Model file for the job. Use its own axes, mm. A direction names the side the tool comes from. Coordinates: 2 decimals unless noted, no trailing zeros. Write each loop counter-clockwise with the first axis right and the second up, starting at its lowest first coordinate (ties: lowest second). Pieces come first, ordered by that corner, then holes.
Q1. Pull direction Y, two halves, no side cores. Call faces 5 (the flat face through (-10, -373.999, 48)), 6 (the flat face through (-10, -384.162, 52)), 7 (the flat face through (336, 19.556, 11)): released by +Y, released by -Y, zero draft, split by the parting line, or undercut.
Q2. Band-saw the part on D-D, the plane y = -91.5. Write the cut outline in (x, z).
Q3. Band-saw the part on C-C, the plane x = 169. Write the cut outline in (y, z), plus the area to 3 significant figures.
Q4. Band-saw the part on B-B, the plane z = 39.5. Write the cut outline in (x, y).
Q5. Which spindle directions (+Z, -Z, +X, -X, +Y, -Y) get a long thin tool onto all of the face, cutting with end or side? Do faces 1 (the flat face through (-10, -258.917, 48)), 2 (the flat face through (0.891, -317, 73)), 3 (the flat face through (-10, -248.426, 52)), 4 (the flat face through (-20.109, -317, 73)). Say none if no direction does.
Q6. Band-saw the part on A-A, the plane y = -351. Write the cut outline in (x, z).
Q7. Pin check, flat tips, straight feed: P1, Ø5, axis at x = -12, z = 46.5, coming from the -Y side; P2, Ø6, axis at y = -361, z = 69.5, coming from the -X side; P3, Ø6, axis at x = 236, y = -295.5, coming from the +Z side; P4, Ø2, axis at x = 62, z = 22, coming from the +Y side. Stop position of each tip, or through.
Q8. Drill centre lines: probe 1 along Z at (x, y) = (315.5, -554); probe 2 along Y at (x, z) = (234, 7); probe 3 along Y at (x, z) = (-20, 18). Where is each one in solid material? Low to high.
from build123d import *

# Parameters (mm, degrees)
SKETCH1_W            = 390
SKETCH1_H            = 756.8
BOSS_EXTRUDE1_DEPTH  = 20
SKETCH2_R            = 6.05
BOSS_EXTRUDE2_DEPTH  = 10
BOSS_EXTRUDE3_START  = 10
SKETCH3_R            = 6.05
BOSS_EXTRUDE3_DEPTH  = 10
CHAMFER1_SIZE        = 10
BOSS_EXTRUDE4_DEPTH  = 50
SKETCH5_W            = 30
SKETCH5_H            = 160
CUT_EXTRUDE1_DEPTH   = 131
CHAMFER2_SIZE        = 10
CUT_EXTRUDE2_DEPTH   = 78
SKETCH7_W            = 25
SKETCH7_H            = 25
BOSS_EXTRUDE5_DEPTH  = 8
FILLET1_R            = 2
FILLET2_R            = 2
SKETCH8_W            = 21
SKETCH8_H            = 10.491742635
SKETCH8_H_2          = 10.163875677
BOSS_EXTRUDE6_DEPTH  = 40
SKETCH9_W            = 21
SKETCH9_H            = 135.736920339
BOSS_EXTRUDE7_DEPTH  = 10
FILLET3_R            = 2
FILLET4_R            = 2
SKETCH15_R           = 7.5
BOSS_EXTRUDE17_DEPTH = 20
SKETCH17_R           = 7.5
CUT_EXTRUDE7_DEPTH   = 10
SKETCH18_R           = 6.05
BOSS_EXTRUDE18_DEPTH = 20


with BuildPart() as part:
    # Sketch1 → Boss-Extrude1 (new body)
    with BuildSketch(Plane.XY):
        with Locations((147.890593688, -358.84384058)):
            Rectangle(SKETCH1_W, SKETCH1_H)
    extrude(amount=BOSS_EXTRUDE1_DEPTH)

    # Sketch2 → Boss-Extrude2 (add)
    with BuildSketch(Plane(origin=(0, 19.55615942, 0), x_dir=(1, 0, 0), z_dir=(0, 1, 0))):
        with Locations(Location((329.77827945, -10, 0), (0, 0, 90))):
            Circle(SKETCH2_R)
    extrude(amount=BOSS_EXTRUDE2_DEPTH)

    # Sketch3 → Boss-Extrude3 (add)
    with BuildSketch(Plane.XZ.offset(737.24384058).offset(BOSS_EXTRUDE3_START)):
        with Locations(Location((329.77827945, 10, 0), (0, 0, 270))):
            Circle(SKETCH3_R)
    extrude(amount=-BOSS_EXTRUDE3_DEPTH)

    # Chamfer1
    # the kernel refuses this chamfer: 10 mm, written as the material it takes off along each edge
    with BuildSketch(Plane(origin=(368.607423567, -737.24384058, 0), x_dir=(0, 0.9996219169112968, -0.027495876610586487), z_dir=(-1, 0, 0))) as chamfer1_piece_1_section:
        Polygon((CHAMFER1_SIZE * 0.999621916911, -CHAMFER1_SIZE * 0.0274958766106), (-CHAMFER1_SIZE * 0.0274958766106, -CHAMFER1_SIZE * 0.999621916911), (0, 0), align=None)
    chamfer1_piece_1 = extrude(amount=441.433659759, mode=Mode.PRIVATE)
    chamfer1_piece_1 = chamfer1_piece_1 - Plane(origin=(329.77827945, -733.933944157, 10), x_dir=(0, 0, -1), z_dir=(0, -1, 0)) * Cylinder(6.05, 923, mode=Mode.PRIVATE)
    add(chamfer1_piece_1, mode=Mode.SUBTRACT)
    with BuildSketch(Plane(origin=(-47.109406312, -762.960670459, 0), x_dir=(-0.027495876610586317, 0, 0.9996219169112968), z_dir=(0, 1, 0)), Plane(origin=(342.890593688, 45.2729893, 20), x_dir=(-0.9996219169112968, 0, 0.027495876610586282), z_dir=(0, -1, 0))) as chamfer1_piece_2:
        Polygon((CHAMFER1_SIZE * 0.999621916911, CHAMFER1_SIZE * 0.0274958766106), (-CHAMFER1_SIZE * 0.0274958766106, CHAMFER1_SIZE * 0.999621916911), (0, 0), align=None)
    extrude(amount=808.233659759, mode=Mode.SUBTRACT)
    with BuildSketch(Plane(origin=(-72.826236192, 19.55615942, 0), x_dir=(0, 0.027495876610586317, 0.9996219169112968), z_dir=(1, 0, 0))) as chamfer1_piece_3_section:
        Polygon((CHAMFER1_SIZE * 0.999621916911, CHAMFER1_SIZE * 0.0274958766106), (-CHAMFER1_SIZE * 0.0274958766106, CHAMFER1_SIZE * 0.999621916911), (0, 0), align=None)
    chamfer1_piece_3 = extrude(amount=441.433659759, mode=Mode.PRIVATE)
    chamfer1_piece_3 = chamfer1_piece_3 - Plane(origin=(329.77827945, 16.24626296, 10), x_dir=(0, 0, -1), z_dir=(0, -1, 0)) * Cylinder(6.05, 923, mode=Mode.PRIVATE)
    add(chamfer1_piece_3, mode=Mode.SUBTRACT)
    with BuildSketch(Plane(origin=(342.890593688, 45.2729893, 0), x_dir=(-0.9996219169112968, 0, -0.027495876610586334), z_dir=(0, -1, 0)), Plane(origin=(-47.109406312, -762.960670459, 20), x_dir=(-0.027495876610586317, 0, -0.9996219169112968), z_dir=(0, 1, 0))) as chamfer1_piece_4:
        Polygon((CHAMFER1_SIZE * 0.999621916911, -CHAMFER1_SIZE * 0.0274958766106), (-CHAMFER1_SIZE * 0.0274958766106, -CHAMFER1_SIZE * 0.999621916911), (0, 0), align=None)
    extrude(amount=808.233659759, mode=Mode.SUBTRACT)
    with BuildSketch(Plane(origin=(368.607423567, -737.24384058, 20), x_dir=(0, 0.9996219169112968, 0.02749587661058643), z_dir=(-1, 0, 0))) as chamfer1_piece_5_section:
        Polygon((CHAMFER1_SIZE * 0.999621916911, CHAMFER1_SIZE * 0.0274958766106), (-CHAMFER1_SIZE * 0.0274958766106, CHAMFER1_SIZE * 0.999621916911), (0, 0), align=None)
    chamfer1_piece_5 = extrude(amount=441.433659759, mode=Mode.PRIVATE)
    chamfer1_piece_5 = chamfer1_piece_5 - Plane(origin=(329.77827945, -733.933944133, 10), x_dir=(0, 0, -1), z_dir=(0, -1, 0)) * Cylinder(6.05, 923, mode=Mode.PRIVATE)
    add(chamfer1_piece_5, mode=Mode.SUBTRACT)
    with BuildSketch(Plane(origin=(-72.826236192, 19.55615942, 20), x_dir=(0, 0.027495876610586317, -0.9996219169112968), z_dir=(1, 0, 0))) as chamfer1_piece_6_section:
        Polygon((CHAMFER1_SIZE * 0.999621916911, -CHAMFER1_SIZE * 0.0274958766106), (-CHAMFER1_SIZE * 0.0274958766106, -CHAMFER1_SIZE * 0.999621916911), (0, 0), align=None)
    chamfer1_piece_6 = extrude(amount=441.433659759, mode=Mode.PRIVATE)
    chamfer1_piece_6 = chamfer1_piece_6 - Plane(origin=(329.77827945, 16.246262993, 10), x_dir=(0, 0, -1), z_dir=(0, -1, 0)) * Cylinder(6.05, 923, mode=Mode.PRIVATE)
    add(chamfer1_piece_6, mode=Mode.SUBTRACT)

    # Sketch4 → Boss-Extrude4 (add)
    with BuildSketch(Plane.XY.offset(20)):
        Polygon((12.890593688, -358.84384058), (12.890593688, -258.84384058), (-37.109406312, -258.84384058), (-37.109406312, -458.84384058), (12.890593688, -458.84384058), align=None)
    extrude(amount=BOSS_EXTRUDE4_DEPTH)

    # Sketch5 → Cut-Extrude1 (cut)
    with BuildSketch(Plane.ZY.offset(37.109406312)):
        with Locations((35, -358.84384058)):
            Rectangle(SKETCH5_W, SKETCH5_H)
    extrude(amount=-CUT_EXTRUDE1_DEPTH, mode=Mode.SUBTRACT)

    # Chamfer2
    chamfer2_edges = [part.edges().sort_by_distance(p)[0] for p in [
        (-37.109406312, -458.84384058, 45),
        (12.890593688, -458.84384058, 45),
        (12.890593688, -258.84384058, 45),
        (-37.109406312, -258.84384058, 45),
        (-12.109406312, -458.84384058, 70),
        (12.890593688, -358.84384058, 70),
        (-12.109406312, -258.84384058, 70),
        (-37.109406312, -358.84384058, 70),
    ]]
    chamfer(chamfer2_edges, length=CHAMFER2_SIZE)

    # Sketch6 → Cut-Extrude2 (cut)
    with BuildSketch(Plane.XY.offset(20)):
        Polygon((-37.109406312, -268.84384058), (-27.109406312, -258.84384058), (2.890593688, -258.84384058), (12.890593688, -268.84384058), (12.890593688, -448.84384058), (2.890593688, -458.84384058), (-27.109406312, -458.84384058), (-37.109406312, -448.84384058), align=None)
    extrude(amount=CUT_EXTRUDE2_DEPTH, mode=Mode.SUBTRACT)

    # Sketch7 → Boss-Extrude5 (add)
    with BuildSketch(Plane.XY.offset(20)):
        with Locations((-9.609406312, -252.94384058)):
            Rectangle(SKETCH7_W, SKETCH7_H)
        with Locations((-9.609406312, -377.94384058)):
            Rectangle(SKETCH7_W, SKETCH7_H)
    extrude(amount=BOSS_EXTRUDE5_DEPTH)

    # Fillet1
    fillet1_edges = [part.edges().sort_by_distance(p)[0] for p in [
        (-9.609406312, -265.44384058, 20),
        (-22.109406312, -252.94384058, 28),
        (2.890593688, -252.94384058, 28),
        (-9.609406312, -240.44384058, 28),
    ]]
    fillet(fillet1_edges, radius=FILLET1_R)

    # Fillet2
    fillet2_edges = [part.edges().sort_by_distance(p)[0] for p in [
        (-22.109406312, -377.94384058, 28),
        (-9.609406312, -390.44384058, 28),
        (2.890593688, -377.94384058, 28),
        (-9.609406312, -365.44384058, 28),
    ]]
    fillet(fillet2_edges, radius=FILLET2_R)

    # Sketch8 → Boss-Extrude6 (add)
    with BuildSketch(Plane.XY.offset(28)):
        with Locations((-9.609406312, -253.671430769)):
            Rectangle(SKETCH8_W, SKETCH8_H)
        with Locations((-9.609406312, -379.080541951)):
            Rectangle(SKETCH8_W, SKETCH8_H_2)
    extrude(amount=BOSS_EXTRUDE6_DEPTH)

    # Sketch9 → Boss-Extrude7 (add)
    with BuildSketch(Plane.XY.offset(68)):
        with Locations((-9.609406312, -316.294019621)):
            Rectangle(SKETCH9_W, SKETCH9_H)
    extrude(amount=BOSS_EXTRUDE7_DEPTH)

    # Fillet3
    fillet3_edges = [part.edges().sort_by_distance(p)[0] for p in [
        (-20.109406312, -316.457953099, 68),
        (0.890593688, -316.457953099, 68),
        (-20.109406312, -316.294019621, 78),
        (0.890593688, -316.294019621, 78),
    ]]
    fillet(fillet3_edges, radius=FILLET3_R)

    # Fillet4
    fillet4_edges = [part.edges().sort_by_distance(p)[0] for p in [
        (0.30480725, -248.425559451, 77.414213562),
        (-9.609406312, -248.425559451, 78),
        (-19.523619875, -248.425559451, 77.414213562),
        (0.30480725, -384.16247979, 77.414213562),
        (-19.523619875, -384.16247979, 77.414213562),
        (0.890593688, -258.917302086, 49),
        (0.890593688, -248.425559451, 52),
        (-20.109406312, -248.425559451, 52),
        (-20.109406312, -258.917302086, 49),
        (0.890593688, -373.998604113, 49),
        (-20.109406312, -373.998604113, 49),
        (-9.609406312, -384.16247979, 78),
        (0.890593688, -384.16247979, 52),
        (-20.109406312, -384.16247979, 52),
    ]]
    fillet(fillet4_edges, radius=FILLET4_R)

    # Sketch15 → Boss-Extrude17 (add)
    with BuildSketch(Plane(origin=(0, 29.55615942, 0), x_dir=(1, 0, 0), z_dir=(0, 1, 0))):
        with Locations(Location((329.77827945, -10, 0), (0, 0, 270))):
            Circle(SKETCH15_R)
    extrude(amount=-BOSS_EXTRUDE17_DEPTH)

    # Sketch17 → Cut-Extrude7 (cut)
    with BuildSketch(Plane(origin=(0, 29.55615942, 0), x_dir=(1, 0, 0), z_dir=(0, 1, 0))):
        with Locations((329.77827945, -10)):
            Circle(SKETCH17_R)
    extrude(amount=-CUT_EXTRUDE7_DEPTH, mode=Mode.SUBTRACT)

    # Sketch18 → Boss-Extrude18 (add)
    with BuildSketch(Plane(origin=(0, 19.55615942, 0), x_dir=(1, 0, 0), z_dir=(0, 1, 0))):
        with Locations(Location((329.77827945, -10, 0), (0, 0, 180))):
            Circle(SKETCH18_R)
    extrude(amount=BOSS_EXTRUDE18_DEPTH)


solid = part.part
Answer sheet:
1. face 5: undercut
1. face 6: released by -Y
1. face 7: released by +Y
2. outline: (-47.11, 10) - (-37.11, 0) - (332.89, 0) - (342.89, 10) - (332.89, 20) - (-37.11, 20) - close
3. outline: (-737.24, 10) - (-727.24, 0) - (9.56, 0) - (19.56, 10) - (9.56, 20) - (-727.24, 20) - close
3. area: 14,900 mm2
4. outline: (-20.11, -382.16) arc R2 ccw to (-18.11, -384.16) - (-1.11, -384.16) arc R2 ccw to (0.89, -382.16) - (0.89, -376) arc R2 ccw to (-1.11, -374) - (-18.11, -374) arc R2 ccw to (-20.11, -376) - close; (-20.11, -256.92) arc R2 ccw to (-18.11, -258.92) - (-1.11, -258.92) arc R2 ccw to (0.89, -256.92) - (0.89, -250.43) arc R2 ccw to (-1.11, -248.43) - (-18.11, -248.43) arc R2 ccw to (-20.11, -250.43) - close
5. face 1: +X, -X
5. face 2: +Z, +X, +Y, -Y
5. face 3: +Z, +X, -X, +Y
5. face 4: +Z, -X, +Y, -Y
6. outline: (-47.11, 10) - (-37.11, 0) - (332.89, 0) - (342.89, 10) - (332.89, 20) - (-37.11, 20) - close; (-20.11, 70) arc R2 ccw to (-18.11, 68) - (-1.11, 68) arc R2 ccw to (0.89, 70) - (0.89, 76) arc R2 ccw to (-1.11, 78) - (-18.11, 78) arc R2 ccw to (-20.11, 76) - close
7. P1: stops at y = -384.16
7. P2: stops at x = -20.11
7. P3: stops at z = 20
7. P4: passes through
8. probe 1: z = 0 to 20
8. probe 2: y = -734.24 to 16.56
8. probe 3: y = -729.24 to 11.56
